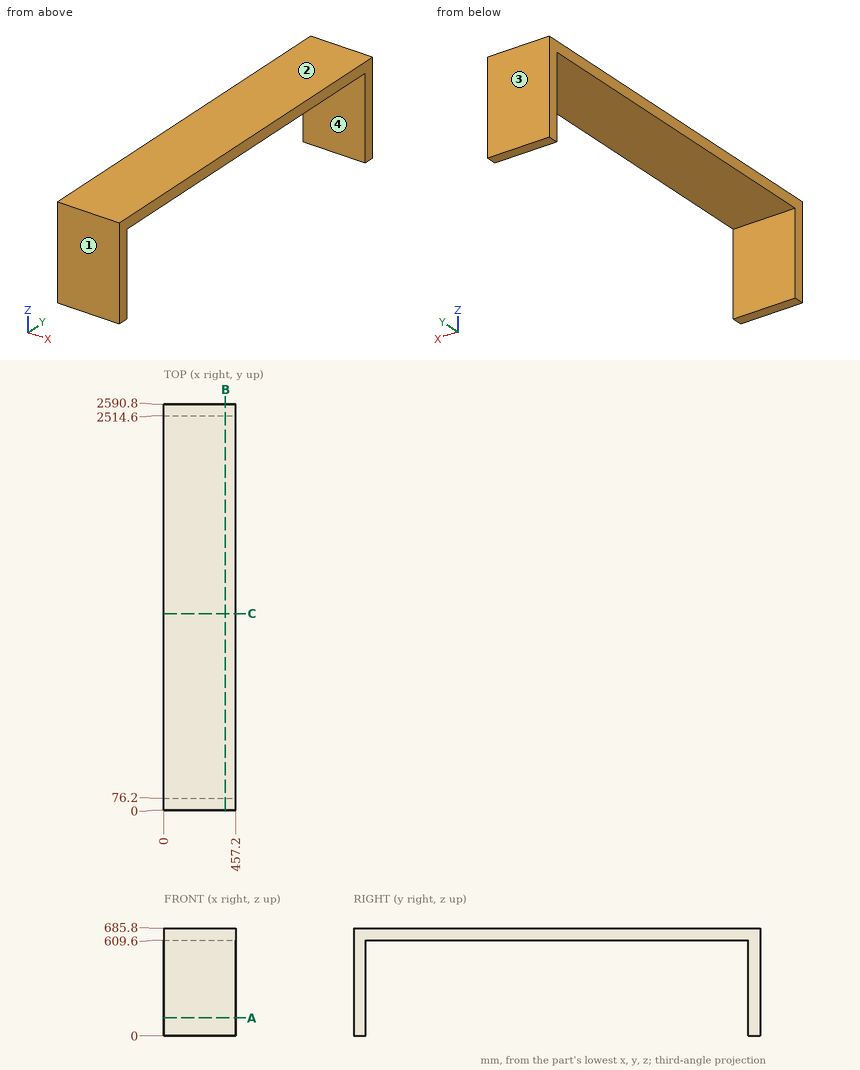
For this review, use the dimensioned drawing (mm, ordinates from the lowest corner) and the shaded views. Give positions to 0.01 mm unless a question says otherwise; leave off trailing zeros. Write each loop counter-clockwise with the first axis right and the second up, starting at its lowest first coordinate (ties: lowest second). Pieces come first, ordered by that corner, then holes.
(1) Consider section B-B, the plane x = 392. Give the boundary of the cut face in (y, z).
(2) To check wall thickness, follow L1, parallel to Y at x = 312, z = 379.5; L2, parallel to Z at x = 354, y = 152.5. State the ranges of each line that lie inside material, in increasing order.
(3) For P1, Ø3, axis at x = 337.5, y = 571, coming from the -Z side, flat-tipped, find the tip position at first contact; note if it passes through.
(4) Consider section A-A, the plane z = 116. Give the boundary of the cut face in (x, y).
(5) Consider section C-C, the plane y = 1255. Give the boundary of the cut face in (x, z), and give its area (3 significant figures).
(6) The part is to be moulded in two halves that separate along Y. For the marked faces 1, 2, 3 and 4, say which applies: released by +Y, released by -Y, zero draft, split by the parting line, or undercut.
Returned:
1. outline: (0, 0) - (76.2, 0) - (76.2, 609.6) - (2514.6, 609.6) - (2514.6, 0) - (2590.8, 0) - (2590.8, 685.8) - (0, 685.8) - close
2. L1: y = 0 to 76.2, 2514.6 to 2590.8
2. L2: z = 609.6 to 685.8
3. P1: stops at z = 609.6
4. outline: (0, 0) - (457.2, 0) - (457.2, 76.2) - (0, 76.2) - close; (0, 2514.6) - (457.2, 2514.6) - (457.2, 2590.8) - (0, 2590.8) - close
5. outline: (0, 609.6) - (457.2, 609.6) - (457.2, 685.8) - (0, 685.8) - close
5. area: 34,800 mm2
6. face 1: released by -Y
6. face 2: zero draft
6. face 3: released by +Y
6. face 4: undercut
